The model under review builds one solid part; all positions refer to its coordinate system, in mm. A direction names the side the tool comes from. Round coordinates to 2 decimals unless told otherwise and drop trailing zeros. Order: outer loops, then holes, each group sorted by start corner. A loop starts at its lowest first (then second) coordinate and runs counter-clockwise, first axis right, second up. Notation, with made-up numbers: M 53.25,46 L 68.25,46 A33 cw 68.25,76 Z; hole C 12.25,26.25 d6. An arc over 180 degrees is marked long. Answer as CSV lines item,"result". Start each with the question number.
from build123d import *

# Parameters (mm, degrees)
F0_R     = 3
F1_DEPTH = 2.5
F2_R     = 0.5


with BuildPart() as f1:
    # F0 (on Top) → F1 (new body)
    with BuildSketch(Plane.XY):
        with BuildLine():
            Line((9.95, 8.746857), (21.08705, 15.176835))
            ThreePointArc((21.08705, 15.176835), (20.351653, 16.14962), (19.571419, 17.086824))
            ThreePointArc((19.571419, 17.086824), (10, 17.320508), (5.011914, 25.492758))
            ThreePointArc((5.011914, 25.492758), (3.810154, 25.699858), (2.6, 25.850338))
            Line((2.6, 25.850338), (2.6, 12.990381))
            ThreePointArc((2.6, 12.990381), (0, 10.390381), (-2.6, 12.990381))
            Line((-2.6, 12.990381), (-2.6, 25.850338))
            ThreePointArc((-2.6, 25.850338), (-3.810154, 25.699858), (-5.011914, 25.492758))
            ThreePointArc((-5.011914, 25.492758), (-10, 17.320508), (-19.571419, 17.086824))
            ThreePointArc((-19.571419, 17.086824), (-20.351653, 16.14962), (-21.08705, 15.176835))
            Line((-21.08705, 15.176835), (-9.95, 8.746857))
            ThreePointArc((-9.95, 8.746857), (-8.998334, 5.195191), (-12.55, 4.243524))
            Line((-12.55, 4.243524), (-23.68705, 10.673503))
            ThreePointArc((-23.68705, 10.673503), (-24.161807, 9.550239), (-24.583333, 8.405934))
            ThreePointArc((-24.583333, 8.405934), (-20, 0), (-24.583333, -8.405934))
            ThreePointArc((-24.583333, -8.405934), (-24.161807, -9.550239), (-23.68705, -10.673503))
            Line((-23.68705, -10.673503), (-12.55, -4.243524))
            ThreePointArc((-12.55, -4.243524), (-8.998334, -5.195191), (-9.95, -8.746857))
            Line((-9.95, -8.746857), (-21.08705, -15.176835))
            ThreePointArc((-21.08705, -15.176835), (-20.351653, -16.14962), (-19.571419, -17.086824))
            ThreePointArc((-19.571419, -17.086824), (-10, -17.320508), (-5.011914, -25.492758))
            ThreePointArc((-5.011914, -25.492758), (-3.810154, -25.699858), (-2.6, -25.850338))
            Line((-2.6, -25.850338), (-2.6, -12.990381))
            ThreePointArc((-2.6, -12.990381), (0, -10.390381), (2.6, -12.990381))
            Line((2.6, -12.990381), (2.6, -25.850338))
            ThreePointArc((2.6, -25.850338), (3.810154, -25.699858), (5.011914, -25.492758))
            ThreePointArc((5.011914, -25.492758), (10, -17.320508), (19.571419, -17.086824))
            ThreePointArc((19.571419, -17.086824), (20.351653, -16.14962), (21.08705, -15.176835))
            Line((21.08705, -15.176835), (9.95, -8.746857))
            ThreePointArc((9.95, -8.746857), (8.998334, -5.195191), (12.55, -4.243524))
            Line((12.55, -4.243524), (23.68705, -10.673503))
            ThreePointArc((23.68705, -10.673503), (24.161807, -9.550239), (24.583333, -8.405934))
            ThreePointArc((24.583333, -8.405934), (20, 0), (24.583333, 8.405934))
            ThreePointArc((24.583333, 8.405934), (24.161807, 9.550239), (23.68705, 10.673503))
            Line((23.68705, 10.673503), (12.55, 4.243524))
            ThreePointArc((12.55, 4.243524), (8.998334, 5.195191), (9.95, 8.746857))
        make_face()
        Circle(F0_R, mode=Mode.SUBTRACT)
    extrude(amount=F1_DEPTH)

    # F2
    f2_edges = [f1.edges().sort_by_distance(p)[0] for p in [
        (23.68705, -10.673503, 1.25),
        (21.08705, -15.176835, 1.25),
        (24.583333, -8.405934, 1.25),
        (19.571419, -17.086824, 1.25),
        (5.011914, -25.492758, 1.25),
        (2.6, -25.850338, 1.25),
        (-2.6, -25.850338, 1.25),
        (-5.011914, -25.492758, 1.25),
        (-21.08705, -15.176835, 1.25),
        (-19.571419, -17.086824, 1.25),
        (-23.68705, -10.673503, 1.25),
        (-24.583333, -8.405934, 1.25),
        (-23.68705, 10.673503, 1.25),
        (-24.583333, 8.405934, 1.25),
        (-21.08705, 15.176835, 1.25),
        (-19.571419, 17.086824, 1.25),
        (-5.011914, 25.492758, 1.25),
        (-2.6, 25.850338, 1.25),
        (2.6, 25.850338, 1.25),
        (5.011914, 25.492758, 1.25),
        (21.08705, 15.176835, 1.25),
        (19.571419, 17.086824, 1.25),
        (23.68705, 10.673503, 1.25),
        (24.583333, 8.405934, 1.25),
    ]]
    fillet(f2_edges, radius=F2_R)


solid = f1.part
Item 1: Wall thickness on probe 1 along X at (y, z) = (-10, 0.85); probe 2 along Y at (x, z) = (0, 1.05); probe 3 along Y at (x, z) = (-12, 2): over which ranges is each line inside the solid? List them lowest first. Write a range as [from, to].
Item 2: Consider section B-B (x = -1.5). State the section outline as (y, z) points.
Item 3: Tool access review of faces 1 (the flat face through (2.6, 19, 1)), 2 (the cylindrical face through (-20.304, -16.21, 1.232)), 3 (the flat face through (15.351, -11.865, 1.232)): name each direction out of +Z, -Z, +X, -X, +Y, -Y from which nothing blocks a thin tool from reaching the whole face with its end or side.
Item 4: Consider section A-A (y = 0). State the section outline as (x, z) points.
Item 5: Consider section C-C (x = 11.25). State the section outline as (y, z) points, and give its area (3 significant figures).
Item 6: The part is to be moulded in two halves that separate along X. For faces 4 (the flat face through (5, 0, 2.5)), 5 (the cylindrical face through (-0.06, -10.39, 1.23)), 6 (the cylindrical face through (20, 0, 1)), say which applies: +X half, -X half, draft (parallel to the pull), parting line (faces both ways), or undercut.
Item 7: For pin 1 (0.8 mm diameter, centred on y = -17.5, z = 1.5, fed in from -X), flat-tipped, find the tip position at first contact; note if it passes through.
Reported:
1,probe 1,"x = [-23.98, -22.52], [-12.12, 12.12], [22.52, 23.98]"
1,probe 2,"y = [-10.39, -3], [3, 10.39]"
1,probe 3,"y = [-16.44, -9.93], [-4.01, 4.01], [9.93, 16.44]"
2,outline,"M -10.87,0 L -2.6,0 L -2.6,2.5 L -10.87,2.5 Z; M 2.6,0 L 10.87,0 L 10.87,2.5 L 2.6,2.5 Z"
3,face 1,"+Z, -Z, +Y"
3,face 2,"+Z, -Z, -X, -Y"
3,face 3,"+Z, -Z"
4,outline,"M -20,0 L -3,0 L -3,2.5 L -20,2.5 Z; M 3,0 L 20,0 L 20,2.5 L 3,2.5 Z"
5,outline,"M -16.71,0 L -9.5,0 L -9.5,2.5 L -16.71,2.5 Z; M -3.9,0 L 3.9,0 L 3.9,2.5 L -3.9,2.5 Z; M 9.5,0 L 16.71,0 L 16.71,2.5 L 9.5,2.5 Z"
5,area,"55.5 mm²"
6,face 4,"draft"
6,face 5,"undercut"
6,face 6,"+X half"
7,pin 1,"stops at x = -10.4"
